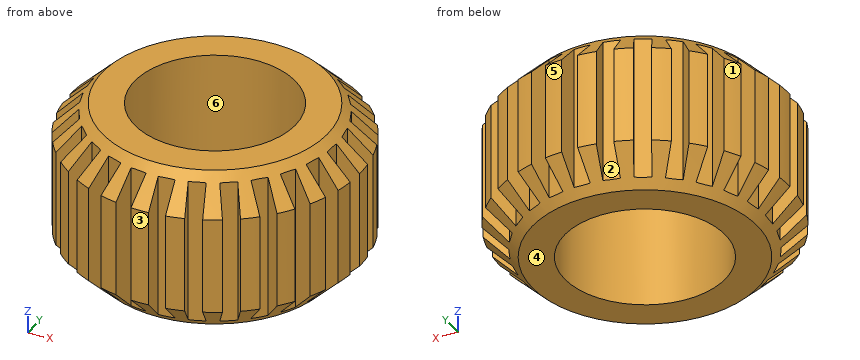
from build123d import *

# Parameters (mm, degrees)
SKETCH1_R           = 9
SKETCH1_R_2         = 5
BOSS_EXTRUDE1_DEPTH = 10
CHAMFER1_SIZE       = 2
CUT_EXTRUDE1_DEPTH  = 11
CIRPATTERN1_COUNT   = 27


with BuildPart() as part:
    # Sketch1 → Boss-Extrude1 (new body)
    with BuildSketch(Plane.XY):
        Circle(SKETCH1_R)
        Circle(SKETCH1_R_2, mode=Mode.SUBTRACT)
    extrude(amount=BOSS_EXTRUDE1_DEPTH)

    # Chamfer1
    chamfer1_edges = [part.edges().sort_by_distance(p)[0] for p in [
        (-9, 0, 10),
        (-9, 0, 0),
    ]]
    chamfer(chamfer1_edges, length=CHAMFER1_SIZE)

    # Sketch2 → Cut-Extrude1 (cut, through all)
    with BuildSketch(Plane.XY):
        with BuildLine():
            Line((-0.5, 7.5), (0.5, 7.5))
            Line((0.5, 7.5), (0.5, 8.986100378))
            ThreePointArc((0.5, 8.986100378), (0, 9), (-0.5, 8.986100378))
            Line((-0.5, 8.986100378), (-0.5, 7.5))
        make_face()
    cut_extrude1 = extrude(amount=CUT_EXTRUDE1_DEPTH, mode=Mode.SUBTRACT)

    # CirPattern1: Cut-Extrude1 ×27 about axis
    cirpattern1_axis = Axis((0, 0, 0), (0, 0, 1))
    for i in range(1, CIRPATTERN1_COUNT):
        add(cut_extrude1.rotate(cirpattern1_axis, i * 360 / CIRPATTERN1_COUNT), mode=Mode.SUBTRACT)


solid = part.part
Input: part model. Units: mm. Frame: model coordinates. Face numbers are marked on the shaded views. A direction names the side the tool comes from. Give positions to 0.01 mm unless a question says otherwise; leave off trailing zeros. Order: outer loops, then holes, each group sorted by start corner. A loop starts at its lowest first (then second) coordinate and runs counter-clockwise, first axis right, second up. Notation, with made-up numbers: (87, -29) - (99, -29) arc R17 cw to (99, -21) - close; hole circle Ø7 at (-12, -10). An arc over 180 degrees is marked (long way). Write each question's results on one line, items separated by ' | '.
Item 1: Material intervals for line 1 along Y through (x, z) = (0, 2.5); line 2 along Y through (x, z) = (7, 8.5); line 3 along Y through (x, z) = (-7.75, 4.25), sorted ascending.
A:
line 1: y = -9 to -5, 5 to 7.5 | line 2: y = -4.82 to -4.62, -3.46 to 2.71, 3.56 to 4.59 | line 3: y = -3.9 to -2.84, -1.8 to -0.95, 0.05 to 0.86, 1.87 to 2.8, 3.89 to 4.58
Item 2: Contact query for flat-ended pins moving along their axis: pin 1 Ø1 at (x, z) = (5, 7.5) entering from +Y; pin 2 Ø5 at (x, y) = (-1.5, -6.5) entering from -Z; pin 3 Ø6 at (x, z) = (6.5, 8) entering from -Y; pin 4 Ø1.6 at (y, z) = (8.5, 5) entering from +X. Output: stop coordinate, or through.
A:
pin 1: stops at y = 7.79 | pin 2: stops at z = 0 | pin 3: stops at y = -8.27 | pin 4: stops at x = 4.66
Item 3: Section A-A (x = 0). Return loops of the section in (y, z), and give its area (4 significant figures).
A:
outline: (-9, 2) - (-7, 0) - (-5, 0) - (-5, 10) - (-7, 10) - (-9, 8) - close; (5, 0) - (7, 0) - (7.5, 0.5) - (7.5, 9.5) - (7, 10) - (5, 10) - close | area: 60.75 mm^2
Item 4: Access query for the marked faces 1 and 2. Directions: +Z, -Z, +X, -X, +Y, -Y. A direction counts if a zero-diameter tool reaches every point of the face in a straight line with its end or side. Return the directions, or none.
A:
face 1: +Z, -Z, -X, +Y | face 2: +Z, -Z
Item 5: Draft query along X for the marked faces 3, 4, 5 and 6. Return one class per face: released by +X, released by -X, zero draft, split by the parting line, or undercut.
A:
face 3: split by the parting line | face 4: zero draft | face 5: released by +X | face 6: undercut
